Work out the finished part from the listing and answer in its coordinate system (mm). Face numbers are marked on the shaded views. A direction names the side the tool comes from. Round coordinates to 2 decimals unless told otherwise and drop trailing zeros. Write each loop counter-clockwise with the first axis right and the second up, starting at its lowest first coordinate (ties: lowest second). Pieces come first, ordered by that corner, then holes.
1. Find section A-A (z = 3). Write down the section's boundary in (x, y) (3 decimals), and give its area (3 significant figures).
2. Find section C-C (z = 10). Write down the section's boundary in (x, y), and give its area (3 significant figures).
3. Find section B-B (y = 12). Write down the section's boundary in (x, z).
4. Find section D-D (y = 1). Write down the section's boundary in (x, z), and give its area (3 significant figures).
5. A tool of negligible diameter and unlimited length cuts with its end or side. For the marked faces 4, 5 and 6, from which of +Z, -Z, +X, -X, +Y, -Y can it reach the whole face along a straight path? Write none if from no direction.
6. Determine the mould class of the marked faces 1, 2 and 3 for opening direction Z: pulls with the +Z half, pulls with the -Z half, needs draft (parallel to the pull), parting line crosses it, or undercut.
7. Flat-ended cylindrical pins translate along their axes: pin 1 Ø3.5 at (x, z) = (-0.5, 7) entering from -Y; pin 2 Ø4 at (y, z) = (5.5, 8.5) entering from -X; pin 3 Ø6 at (y, z) = (-14.5, 9.5) entering from -X; pin 4 Ø1.4 at (x, y) = (0, -25.27) entering from +Z. Find the tip coordinate at first contact, or state that the pin passes through.
8. Straight lines are drawn through the part: probe 1 along Y at (x, z) = (0, 11.4); probe 2 along X at (y, z) = (-21, 7.25); probe 3 along Y at (x, z) = (-0.5, 8.5). For each, find the intervals that lie inside material, in ascending order.
```python
from build123d import *

# Parameters (mm, degrees)
F1_DEPTH = 14
F2_W     = 11.5
F2_H     = 2.4
F2_W_2   = 7.4604106426
F2_H_2   = 3.5
F3_DEPTH = 12.5


with BuildPart() as f1:
    # F0 (on Top) → F1 (new body)
    with BuildSketch(Plane.XY):
        with BuildLine():
            Line((3.625, -25.2749305218), (3.6217764293, -25.1220891128))
            ThreePointArc((3.6217764293, -25.1220891128), (0, -21.6499305218), (-3.6217764293, -25.1220891128))
            Line((-3.6217764293, -25.1220891128), (-3.625, -25.2749305218))
            Line((-3.625, -25.2749305218), (-0.75, -25.2749305218))
            ThreePointArc((-0.75, -25.2749305218), (0, -24.5249305218), (0.75, -25.2749305218))
            Line((0.75, -25.2749305218), (3.625, -25.2749305218))
        make_face()
        with BuildLine():
            Line((3.6217764293, -25.1220891128), (2.8, 13.841370428))
            ThreePointArc((2.8, 13.841370428), (0, 11.041370428), (-2.8, 13.841370428))
            Line((-2.8, 13.841370428), (-3.6217764293, -25.1220891128))
            ThreePointArc((-3.6217764293, -25.1220891128), (0, -21.6499305218), (3.6217764293, -25.1220891128))
        make_face()
        with BuildLine():
            Line((0.75, 13.841370428), (2.8, 13.841370428))
            ThreePointArc((2.8, 13.841370428), (0, 16.641370428), (-2.8, 13.841370428))
            Line((-2.8, 13.841370428), (-0.75, 13.841370428))
            ThreePointArc((-0.75, 13.841370428), (0, 14.591370428), (0.75, 13.841370428))
        make_face()
        with BuildLine():
            ThreePointArc((-3.625, -25.2749305218), (0, -28.8999305218), (3.625, -25.2749305218))
            Line((3.625, -25.2749305218), (0.75, -25.2749305218))
            ThreePointArc((0.75, -25.2749305218), (0, -26.0249305218), (-0.75, -25.2749305218))
            Line((-0.75, -25.2749305218), (-3.625, -25.2749305218))
        make_face()
        with BuildLine():
            ThreePointArc((-2.8, 13.841370428), (0, 11.041370428), (2.8, 13.841370428))
            Line((2.8, 13.841370428), (0.75, 13.841370428))
            ThreePointArc((0.75, 13.841370428), (0, 13.091370428), (-0.75, 13.841370428))
            Line((-0.75, 13.841370428), (-2.8, 13.841370428))
        make_face()
    extrude(amount=F1_DEPTH)

    # F2 (on Right) → F3 (cut, symmetric)
    with BuildSketch(Plane.YZ):
        Polygon((-28.9036631584, 17.2806195915), (-28.9036631584, 14.1698746011), (16.6315902025, 12), (16.6315902025, 18.462985754), align=None)
        Polygon((16.6315902025, 2), (-28.9036631584, 0), (16.7194342289, 0), align=None)
        with Locations((17.2709319741, 5.8)):
            Rectangle(F2_W, F2_H)
        with Locations((17.2709319741, 8.2)):
            Rectangle(F2_W, F2_H)
        with Locations((-25.1734578371, 8.75)):
            Rectangle(F2_W_2, F2_H_2)
        with Locations((-25.1734578371, 5.25)):
            Rectangle(F2_W_2, F2_H_2)
    extrude(amount=F3_DEPTH, both=True, mode=Mode.SUBTRACT)


solid = f1.part
```
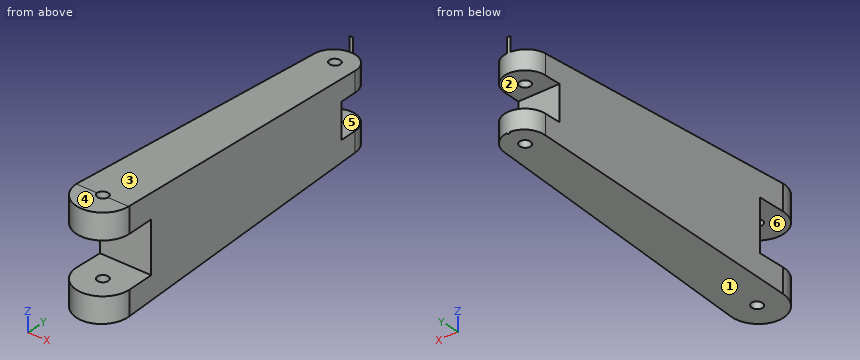
Worked answers:
1. outline: (-3.625, -25.275) arc R3.625 ccw to (3.625, -25.275) - (2.8, 13.841) arc R2.8 ccw to (-2.8, 13.841) - close; hole circle Ø1.5 at (0, -25.275); hole circle Ø1.5 at (0, 13.841)
1. area: 281 mm2
2. outline: (-3.54, -21.44) - (3.54, -21.44) - (2.8, 13.84) arc R2.8 ccw to (-2.8, 13.84) - close; hole circle Ø1.5 at (0, 13.84)
2. area: 234 mm2
3. outline: (-2.84, 1.8) - (2.84, 1.8) - (2.84, 4.6) - (-2.84, 4.6) - close; (-2.84, 9.4) - (2.84, 9.4) - (2.84, 12.22) - (-2.84, 12.22) - close
4. outline: (-3.07, 1.31) - (3.07, 1.31) - (3.07, 12.74) - (-3.07, 12.74) - close
4. area: 70.2 mm2
5. face 4: +Z, +X, -X, +Y, -Y
5. face 5: +X, -X, +Y
5. face 6: +X, -X, -Y
6. face 1: pulls with the -Z half
6. face 2: undercut
6. face 3: pulls with the +Z half
7. pin 1: stops at y = -21.44
7. pin 2: stops at x = -3.02
7. pin 3: stops at x = -3.46
7. pin 4: passes through
8. probe 1: y = -28.9 to -26.02, -24.52 to 13.09, 14.59 to 16.64
8. probe 2: x = -3.53 to 3.53
8. probe 3: y = -21.44 to 11.52
